```python
from build123d import *

# Parameters (mm, degrees)
SKETCH1_W                = 115
SKETCH1_H                = 229
BOSS_EXTRUDE1_DEPTH      = 77
SKETCH12_W               = 26
SKETCH12_H               = 22.5
BOSS_EXTRUDE3_DEPTH      = 5
BOSS_EXTRUDE3_DEPTH_BACK = 83
FILLET2_R                = 15
FILLET3_R                = 15
FILLET4_R                = 2
SKETCH13_R               = 7.5
BOSS_EXTRUDE4_DEPTH      = 6
SKETCH13_6_R             = 16.5
BOSS_EXTRUDE5_DEPTH      = 10
SKETCH14_R               = 8.5
BOSS_EXTRUDE6_DEPTH      = 6
SKETCH15_R               = 2.5
BOSS_EXTRUDE7_DEPTH      = 10


with BuildPart() as part:
    # Sketch1 → Boss-Extrude1 (new body)
    with BuildSketch(Plane(origin=(0, 0, 0), x_dir=(1, 0, 0), z_dir=(0, 1, 0))):
        Rectangle(SKETCH1_W, SKETCH1_H)
    extrude(amount=BOSS_EXTRUDE1_DEPTH)

    # Sketch12 → Boss-Extrude3 (add, two sides)
    with BuildSketch(Plane(origin=(0, 77, 0), x_dir=(1, 0, 0), z_dir=(0, 1, 0))) as boss_extrude3_sk:
        with Locations((-49.5, -108.25)):
            Rectangle(SKETCH12_W, SKETCH12_H)
        with Locations((49.5, -108.25)):
            Rectangle(SKETCH12_W, SKETCH12_H)
        with Locations((49.5, 108.25)):
            Rectangle(SKETCH12_W, SKETCH12_H)
        with Locations((-49.5, 108.25)):
            Rectangle(SKETCH12_W, SKETCH12_H)
    extrude(amount=BOSS_EXTRUDE3_DEPTH)
    extrude(boss_extrude3_sk.sketch, amount=-BOSS_EXTRUDE3_DEPTH_BACK)

    # Fillet2
    fillet2_edges = [part.edges().sort_by_distance(p)[0] for p in [
        (-62.5, 38, -119.5),
        (62.5, 38, -119.5),
        (62.5, 38, 119.5),
        (-62.5, 38, 119.5),
    ]]
    fillet(fillet2_edges, radius=FILLET2_R)

    # Fillet3
    fillet3_edges = [part.edges().sort_by_distance(p)[0] for p in [
        (-36.5, 79.5, -97),
        (-36.5, -3, -97),
        (36.5, 79.5, -97),
        (36.5, -3, -97),
        (36.5, 79.5, 97),
        (36.5, -3, 97),
        (-36.5, 79.5, 97),
        (-36.5, -3, 97),
    ]]
    fillet(fillet3_edges, radius=FILLET3_R)

    # Fillet4
    fillet4_edges = [part.edges().sort_by_distance(p)[0] for p in [
        (-36.5, 38, -119.5),
        (-62.5, 38, -97),
        (36.5, 38, -119.5),
        (62.5, 38, -97),
        (36.5, 38, 119.5),
        (62.5, 38, 97),
        (-36.5, 38, 119.5),
        (-62.5, 38, 97),
    ]]
    fillet(fillet4_edges, radius=FILLET4_R)

    # Sketch13 → Boss-Extrude4 (add)
    with BuildSketch(Plane(origin=(57.5, 0, 0), x_dir=(0, 0, -1), z_dir=(1, 0, 0))):
        with Locations((-25, 18)):
            Circle(SKETCH13_R)
    extrude(amount=BOSS_EXTRUDE4_DEPTH)

    # Sketch13_6 → Boss-Extrude5 (add)
    with BuildSketch(Plane(origin=(57.5, 0, 0), x_dir=(0, 0, -1), z_dir=(1, 0, 0))):
        with Locations((36, 37)):
            Circle(SKETCH13_6_R)
    extrude(amount=BOSS_EXTRUDE5_DEPTH)

    # Sketch14 → Boss-Extrude6 (add)
    with BuildSketch(Plane(origin=(67.5, 0, 0), x_dir=(0, 0, -1), z_dir=(1, 0, 0))):
        with Locations((36, 37)):
            Circle(SKETCH14_R)
    extrude(amount=BOSS_EXTRUDE6_DEPTH)

    # Sketch15 → Boss-Extrude7 (add)
    with BuildSketch(Plane(origin=(73.5, 0, 0), x_dir=(0, 0, -1), z_dir=(1, 0, 0))):
        with Locations((36, 37)):
            Circle(SKETCH15_R)
    extrude(amount=BOSS_EXTRUDE7_DEPTH)


solid = part.part
```
Verification items for the finished model (mm, model axes). A direction names the side the tool comes from. Round coordinates to 2 decimals unless told otherwise and drop trailing zeros. Write each loop counter-clockwise with the first axis right and the second up, starting at its lowest first coordinate (ties: lowest second). Pieces come first, ordered by that corner, then holes. Notation, with made-up numbers: (11.5, 66) -> (66.5, 66) arc R28 ccw to (66.5, 98) -> close; hole circle Ø5 at (-35, 83). An arc over 180 degrees is marked (long way). Write each question's results on one line, items separated by ' | '.
Q1. Sectioned sample at B-B, the plane x = 1.5. Record the boundary of the cut face in (y, z).
Derived:
outline: (0, -114.5) -> (77, -114.5) -> (77, 114.5) -> (0, 114.5) -> close
Q2. Thickness scan on probe 1 along Z at (x, y) = (58, 30); probe 2 along Z at (x, y) = (-2, 71); probe 3 along Y at (x, z) = (21, 23.5). Record the ranges inside material, lowest first.
Derived:
probe 1: z = -115.21 to -97, -50.94 to -21.06, 97 to 115.21 | probe 2: z = -114.5 to 114.5 | probe 3: y = 0 to 77
Q3. Go/stop test with flat-tipped pins: pin 1 Ø6 at (y, z) = (35.5, 102.5) entering from +X; pin 2 Ø10 at (x, z) = (-15.5, -64) entering from -Y; pin 3 Ø4.5 at (x, y) = (54, 56) entering from -Z; pin 4 Ø18.5 at (y, z) = (39.5, -32.5) entering from +X. Record where each tip stops, or that it passes through.
Derived:
pin 1: stops at x = 62.5 | pin 2: stops at y = 0 | pin 3: stops at z = -118.89 | pin 4: stops at x = 83.5
Q4. Sectioned sample at C-C, the plane z = 25. Record the boundary of the cut face in (x, y), and give its area (4 significant figures).
Derived:
outline: (-57.5, 0) -> (57.5, 0) -> (57.5, 10.5) -> (63.5, 10.5) -> (63.5, 25.5) -> (57.5, 25.5) -> (57.5, 77) -> (-57.5, 77) -> close | area: 8,945 mm²
Q5. Draft check along Z on faces 4 (the face through (-1, 77, -2)), 5 (the face through (58.22, 37.38, 114.99)), 6 (the face through (-62.5, 39, 102)). Enter one of: released by +Z, released by -Z, zero draft, split by the parting line, or undercut.
Derived:
face 4: undercut | face 5: released by +Z | face 6: zero draft
Q6. Sectioned sample at A-A, the plane z = -36. Record the boundary of the cut face in (x, y).
Derived:
outline: (-57.5, 0) -> (57.5, 0) -> (57.5, 20.5) -> (67.5, 20.5) -> (67.5, 28.5) -> (73.5, 28.5) -> (73.5, 34.5) -> (83.5, 34.5) -> (83.5, 39.5) -> (73.5, 39.5) -> (73.5, 45.5) -> (67.5, 45.5) -> (67.5, 53.5) -> (57.5, 53.5) -> (57.5, 77) -> (-57.5, 77) -> close
Q7. Access from +Z, -Z, +X, -X, +Y, -Y to the whole of each face (thin tool, end or side, straight path). Record for faces 1 (the face through (-58, 39, 97)), 2 (the face through (-1, 38, 114.5)), 3 (the face through (60.5, 23.1, 30.5)).
Derived:
face 1: -X | face 2: +Z, +Y, -Y | face 3: +X
